For this review, take the finished solid that the model builds, in its own axes (mm). Face numbers are marked on the shaded views. Give positions to 0.01 mm unless a question says otherwise; leave off trailing zeros. Loops run counter-clockwise (first coordinate to the right, second up) from the corner with the lowest first, then second, coordinate; pieces in that order, holes last. Notation, with made-up numbers: (-38, 32.5) -> (-13, 32.5) arc R18 cw to (-13, 55.5) -> close; hole circle Ø1 at (76, 20.5). An arc over 180 degrees is marked (long way). One line per question, with ' | ' between items. Start each with the question number.
(1) Wall thickness on probe 1 along Z at (x, y) = (0.4, 3.45); probe 2 along X at (y, z) = (0.9, 0.5); probe 3 along X at (y, z) = (2.2, -1): over which ranges is each line inside the solid? List them lowest first.
(2) Consider section A-A (z = 0). Write out the cut boundary in (x, y).
(3) Consider section C-C (y = 0.65). Write out the cut boundary in (x, z), and give its area (3 significant figures).
(4) Consider section D-D (x = 1.5). Write out the cut boundary in (y, z), and give its area (3 significant figures).
(5) Insertion check: P1, Ø1.5, axis at x = 1, y = 3.5, coming from the +Z side. The pin has a flat end and moves straight along its axis. Give the tip position at first contact, or say it passes through.
(6) Draft analysis for pull direction X (two halves, no side actions). For the marked faces 1, 2 and 3, state which applies: +X half, -X half, draft (parallel to the pull), parting line (faces both ways), or undercut.
(7) Consider section B-B (x = 0.55). Write out the cut boundary in (y, z), and give its area (3 significant figures).
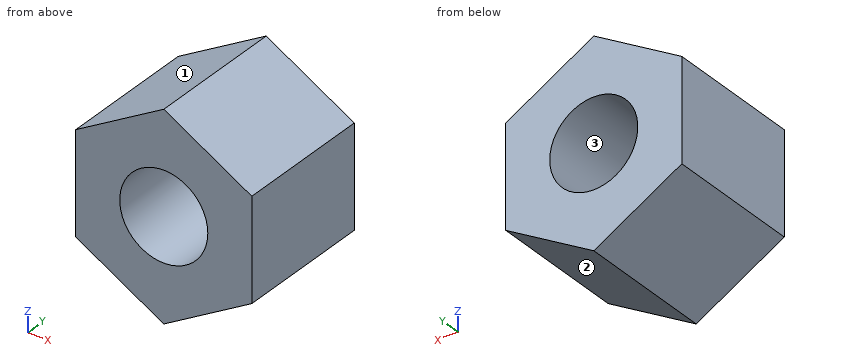
from build123d import *

# Parameters (mm, degrees)
BOSS_EXTRUDE1_DEPTH       = 4
M3X0_5_TAPPED_HOLE1_D     = 2.5
M3X0_5_TAPPED_HOLE1_DEPTH = 13.5
M3X0_5_TAPPED_HOLE1_TIP   = 0.751075774


with BuildPart() as part:
    # Sketch2 → Boss-Extrude1 (new body)
    with BuildSketch(Plane(origin=(0, 0, 0), x_dir=(1, 0, 0), z_dir=(0, 1, 0))):
        Polygon((1.25, 0.721687836), (-2.5, -1.443375673), (0, -2.886751346), (1.666666667, 0), align=None)
        Polygon((0.833333333, 1.443375673), (-2.5, 1.443375673), (-2.5, -1.443375673), (1.25, 0.721687836), align=None)
        Polygon((0.833333333, 1.443375673), (0, 2.886751346), (-2.5, 1.443375673), align=None)
        Polygon((2.5, 1.443375673), (0, 2.886751346), (0.833333333, 1.443375673), align=None)
        Polygon((1.25, 0.721687836), (2.5, 1.443375673), (0.833333333, 1.443375673), align=None)
        Polygon((1.666666667, 0), (2.5, 1.443375673), (1.25, 0.721687836), align=None)
        Polygon((2.5, -1.443375673), (2.5, 1.443375673), (1.666666667, 0), align=None)
        Polygon((0, -2.886751346), (2.5, -1.443375673), (1.666666667, 0), align=None)
    extrude(amount=BOSS_EXTRUDE1_DEPTH)

    # M3x0.5 Tapped Hole1
    with Locations(Plane(origin=(0, 0, 0), x_dir=(-1, 0, 0), z_dir=(0, -1, 0))):
        with Locations((0, 0)):
            Hole(M3X0_5_TAPPED_HOLE1_D / 2, depth=M3X0_5_TAPPED_HOLE1_DEPTH)
            with Locations((0, 0, -(M3X0_5_TAPPED_HOLE1_DEPTH + M3X0_5_TAPPED_HOLE1_TIP / 2))):  # 118° drill point
                Cone(0, M3X0_5_TAPPED_HOLE1_D / 2, M3X0_5_TAPPED_HOLE1_TIP, mode=Mode.SUBTRACT)


solid = part.part
A:
1) probe 1: z = -2.66 to -1.18, 1.18 to 2.66 | probe 2: x = -2.5 to -1.15, 1.15 to 2.5 | probe 3: x = -2.5 to -0.75, 0.75 to 2.5
2) outline: (-2.5, 0) -> (-1.25, 0) -> (-1.25, 4) -> (-2.5, 4) -> close; (1.25, 0) -> (2.5, 0) -> (2.5, 4) -> (1.25, 4) -> close
3) outline: (-2.5, -1.44) -> (0, -2.89) -> (2.5, -1.44) -> (2.5, 1.44) -> (0, 2.89) -> (-2.5, 1.44) -> close; hole circle Ø2.5 at (0, 0) | area: 16.7 mm^2
4) outline: (0, -2.02) -> (4, -2.02) -> (4, 2.02) -> (0, 2.02) -> close | area: 16.2 mm^2
5) P1: stops at z = 2.74
6) face 1: -X half | face 2: +X half | face 3: undercut
7) outline: (0, -2.57) -> (4, -2.57) -> (4, -1.12) -> (0, -1.12) -> close; (0, 1.12) -> (4, 1.12) -> (4, 2.57) -> (0, 2.57) -> close | area: 11.6 mm^2
